```python
from build123d import *

# Parameters (mm, degrees)
SKETCH1_W                     = 17
SKETCH1_H                     = 39
SKETCH1_R                     = 1
SKETCH1_W_2                   = 12
SKETCH1_H_2                   = 23
SERVOBRACKET_DEPTH            = 2.5
SKETCH1_5_W                   = 2.5
SKETCH1_5_H                   = 10
SUPPORTLEGS_DEPTH             = 21.1
SKETCH2_W                     = 2
SKETCH2_H                     = 10
SUPPORTFOOT_DEPTH             = 5
BASEBOLTHOLE_START            = -3
SKETCH3_R                     = 1
BASEBOLTHOLE_DEPTH            = 25.6
SERVONUTSLOTS_DEPTH           = 1
BASENUTSLOTS_DEPTH            = 1
SKETCH6_W                     = 2.5
SKETCH6_H                     = 4
TUBEHOLDERBASE_DEPTH          = 12
SKETCH7_W                     = 4
SKETCH7_H                     = 1
TUBEHOLDERSTIFFENERRIBS_DEPTH = 30.6
SKETCH8_W                     = 1
SKETCH8_H                     = 1
SKETCH8_H_2                   = 0.25
TUBECLIPENTRANCES_DEPTH       = 2
SKETCH9_W                     = 1.5
SKETCH9_H                     = 1.5
TUBECLIPLOCKSLOT_DEPTH        = 0.6
TUBECLIPLOCKSLOT2_DEPTH       = 0.6
SUPPORTLEGEXTENSION_DEPTH     = 10.55
SKETCH8_4_W                   = 0.2
SKETCH8_4_H                   = 1.5
TUBECLIPLOCKCLEARANCE_DEPTH   = 0.5


with BuildPart() as part:
    # Sketch1 → ServoBracket (new body)
    with BuildSketch(Plane.XY):
        with Locations((0, 19.5)):
            Rectangle(SKETCH1_W, SKETCH1_H)
        with Locations((-3.5, 33.5)):
            Circle(SKETCH1_R, mode=Mode.SUBTRACT)
        with Locations((-3.5, 5.5)):
            Circle(SKETCH1_R, mode=Mode.SUBTRACT)
        with Locations((3.5, 5.5)):
            Circle(SKETCH1_R, mode=Mode.SUBTRACT)
        with Locations((3.5, 33.5)):
            Circle(SKETCH1_R, mode=Mode.SUBTRACT)
        with Locations((0, 19.5)):
            Rectangle(SKETCH1_W_2, SKETCH1_H_2, mode=Mode.SUBTRACT)
    extrude(amount=SERVOBRACKET_DEPTH)

    # Sketch1_5 → SupportLegs (add)
    with BuildSketch(Plane.XY):
        with Locations((-7.25, 19.5)):
            Rectangle(SKETCH1_5_W, SKETCH1_5_H)
        with Locations((7.25, 19.5)):
            Rectangle(SKETCH1_5_W, SKETCH1_5_H)
    extrude(amount=-SUPPORTLEGS_DEPTH)

    # Sketch2 → SupportFoot (add)
    with BuildSketch(Plane.ZY.offset(8.5)):
        with Locations((-20.1, 19.5)):
            Rectangle(SKETCH2_W, SKETCH2_H)
    supportfoot = extrude(amount=SUPPORTFOOT_DEPTH)

    # Sketch3 → BaseBoltHole (cut)
    with BuildSketch(Plane.XY.offset(-19.1).offset(BASEBOLTHOLE_START)):
        with Locations((-11, 19.5)):
            Circle(SKETCH3_R)
    basebolthole = extrude(amount=BASEBOLTHOLE_DEPTH, mode=Mode.SUBTRACT)

    # SupportFoot2: SupportFoot, BaseBoltHole across plane
    add(supportfoot.mirror(Plane(origin=(0, 0, 0), x_dir=(0, 0, 1), z_dir=(1, 0, 0))))
    add(basebolthole.mirror(Plane(origin=(0, 0, 0), x_dir=(0, 0, 1), z_dir=(1, 0, 0))), mode=Mode.SUBTRACT)

    # Sketch4 → ServoNutSlots (cut)
    with BuildSketch(Plane.XY.offset(2.5)):
        Polygon((-4.654700538, 7.5), (-2.345299462, 7.5), (-1.190598923, 5.5), (-2.345299462, 3.5), (-4.654700538, 3.5), (-5.809401077, 5.5), align=None)
        Polygon((-1.190598923, 33.5), (-2.345299462, 35.5), (-4.654700538, 35.5), (-5.809401077, 33.5), (-4.654700538, 31.5), (-2.345299462, 31.5), align=None)
        Polygon((2.345299462, 31.5), (1.190598923, 33.5), (2.345299462, 35.5), (4.654700538, 35.5), (5.809401077, 33.5), (4.654700538, 31.5), align=None)
        Polygon((4.654700538, 7.5), (2.345299462, 7.5), (1.190598923, 5.5), (2.345299462, 3.5), (4.654700538, 3.5), (5.809401077, 5.5), align=None)
    extrude(amount=-SERVONUTSLOTS_DEPTH, mode=Mode.SUBTRACT)

    # Sketch5 → BaseNutSlots (cut)
    with BuildSketch(Plane.XY.offset(-19.1)):
        Polygon((-11, 21.809401077), (-13, 20.654700538), (-13, 18.345299462), (-11, 17.190598923), (-9, 18.345299462), (-9, 20.654700538), align=None)
        Polygon((11, 21.809401077), (9, 20.654700538), (9, 18.345299462), (11, 17.190598923), (13, 18.345299462), (13, 20.654700538), align=None)
    extrude(amount=-BASENUTSLOTS_DEPTH, mode=Mode.SUBTRACT)

    # Sketch6 → TubeHolderBase (add)
    with BuildSketch(Plane.XY.offset(2.5)):
        with Locations((-7.25, 21.65)):
            Rectangle(SKETCH6_W, SKETCH6_H)
    tubeholderbase = extrude(amount=TUBEHOLDERBASE_DEPTH)

    # Sketch7 → TubeHolderStiffenerRibs (add)
    with BuildSketch(Plane.XY.offset(14.5)):
        with Locations((-10.5, 23.15)):
            Rectangle(SKETCH7_W, SKETCH7_H)
        with Locations((-10.5, 20.15)):
            Rectangle(SKETCH7_W, SKETCH7_H)
    tubeholderstiffenerribs = extrude(amount=-TUBEHOLDERSTIFFENERRIBS_DEPTH)

    # TubeHolder2: TubeHolderBase, TubeHolderStiffenerRibs across plane
    add(tubeholderbase.mirror(Plane.ZX.offset(13.8)))
    add(tubeholderstiffenerribs.mirror(Plane.ZX.offset(13.8)))

    # Sketch8 → TubeClipEntrances (cut)
    with BuildSketch(Plane.ZY.offset(8.5)):
        with Locations((11.1, 21.65)):
            Rectangle(SKETCH8_W, SKETCH8_H)
        with Locations((11.1, 22.275)):
            Rectangle(SKETCH8_W, SKETCH8_H_2)
        with Locations((11.1, 21.025)):
            Rectangle(SKETCH8_W, SKETCH8_H_2)
        with Locations((10.3, 6.575)):
            Rectangle(SKETCH8_W, SKETCH8_H_2)
        with Locations((10.3, 5.325)):
            Rectangle(SKETCH8_W, SKETCH8_H_2)
        with Locations((10.3, 5.95)):
            Rectangle(SKETCH8_W, SKETCH8_H)
    extrude(amount=-TUBECLIPENTRANCES_DEPTH, mode=Mode.SUBTRACT)

    # Sketch9 → TubeClipLockSlot (cut)
    with BuildSketch(Plane(origin=(0, 0, 11.6), x_dir=(-1, 0, 0), z_dir=(0, 0, -1))):
        with Locations((7.25, 21.65)):
            Rectangle(SKETCH9_W, SKETCH9_H)
    extrude(amount=-TUBECLIPLOCKSLOT_DEPTH, mode=Mode.SUBTRACT)

    # Sketch10 → TubeClipLockSlot2 (cut)
    with BuildSketch(Plane(origin=(0, 0, 10.8), x_dir=(-1, 0, 0), z_dir=(0, 0, -1))):
        Polygon((6.5, 5.45), (6.5, 5.2), (8, 5.2), (8, 6.7), (6.5, 6.7), align=None)
    extrude(amount=-TUBECLIPLOCKSLOT2_DEPTH, mode=Mode.SUBTRACT)

    # Sketch11 → SupportLegExtension (add)
    with BuildSketch(Plane.XZ.offset(-14.5)):
        Polygon((-6, 0), (-8.5, 0), (-8.5, -19.1), (-13.5, -19.1), (-13.5, -21.1), (-6, -21.1), align=None)
    extrude(amount=SUPPORTLEGEXTENSION_DEPTH)

    # Sketch8_4 → TubeClipLockClearance (cut)
    with BuildSketch(Plane.ZY.offset(8.5)):
        with Locations((10.9, 5.95)):
            Rectangle(SKETCH8_4_W, SKETCH8_4_H)
        with Locations((11.7, 21.65)):
            Rectangle(SKETCH8_4_W, SKETCH8_4_H)
    extrude(amount=-TUBECLIPLOCKCLEARANCE_DEPTH, mode=Mode.SUBTRACT)


solid = part.part
```
Work out the finished part from the listing and answer in its coordinate system (mm). A direction names the side the tool comes from. Give positions to 0.01 mm unless a question says otherwise; leave off trailing zeros. Loops run counter-clockwise (first coordinate to the right, second up) from the corner with the lowest first, then second, coordinate; pieces in that order, holes last. Notation, with made-up numbers: (-35, -15) -> (-13, -15) arc R16 cw to (-13, 12) -> close; hole circle Ø9 at (-34, 68). An arc over 180 degrees is marked (long way). Use CSV: the item, a comma, the result in double quotes.
1. The part is cut by section A-A (x = 3.5). Write down the section's boundary in (y, z).
Found:
outline,"(0, 0) -> (4.5, 0) -> (4.5, 1.5) -> (3.5, 1.5) -> (3.5, 2.5) -> (0, 2.5) -> close; (6.5, 0) -> (8, 0) -> (8, 2.5) -> (7.5, 2.5) -> (7.5, 1.5) -> (6.5, 1.5) -> close; (31, 0) -> (32.5, 0) -> (32.5, 1.5) -> (31.5, 1.5) -> (31.5, 2.5) -> (31, 2.5) -> close; (34.5, 0) -> (39, 0) -> (39, 2.5) -> (35.5, 2.5) -> (35.5, 1.5) -> (34.5, 1.5) -> close"
2. Straight lines are drawn through the part: line 1 (Y direction, x = -3.5, z = 0.5); line 2 (X direction, y = 19, z = -20); line 3 (Y direction, x = -11.5, z = 11.5). For each, find the intervals that lie inside material, in ascending order.
Found:
line 1,"0 to 4.5, 6.5 to 8, 31 to 32.5, 34.5 to 39"
line 2,"-13.5 to -13, -9 to -6, 6 to 9, 13 to 13.5"
line 3,"3.95 to 4.95, 6.95 to 7.95, 19.65 to 20.65, 22.65 to 23.65"
3. A tool of negligible diameter and unlimited length cuts with its end or side. For faces 5 (the flat face through (13, 19.5, -19.6)), 6 (the flat face through (-11, 23, -16.1)), 7 (the flat face through (9.7, 19.4, -21.1)), 8 (the flat face through (-10, 7.95, -1)), 9 (the flat face through (-7, 6, 11.4)), from which of +Z, -Z, +X, -X, +Y, -Y can it reach the whole face along a straight path? Write none if from no direction.
Found:
face 5,"+Z"
face 6,"-X, +Y, -Y"
face 7,"-Z, +X, -X, +Y, -Y"
face 8,"+Z, -X"
face 9,"none"
4. The mould has two halves that part along X. Classify faces 1 (the flat face through (3, 35.5, 2)), 2 (the flat face through (-6, 6, 8)), 3 (the flat face through (-13.5, 14, -20)), 4 (the flat face through (-3, 35.5, 2)): +X half, -X half, draft (parallel to the pull), parting line (faces both ways), or undercut.
Found:
face 1,"undercut"
face 2,"+X half"
face 3,"-X half"
face 4,"undercut"
5. The part is cut by section B-B (z = 5). Write down the section's boundary in (x, y), then the cut area to 3 significant figures.
Found:
outline,"(-12.5, 3.95) -> (-6, 3.95) -> (-6, 7.95) -> (-12.5, 7.95) -> (-12.5, 6.95) -> (-8.5, 6.95) -> (-8.5, 4.95) -> (-12.5, 4.95) -> close; (-12.5, 19.65) -> (-6, 19.65) -> (-6, 23.65) -> (-12.5, 23.65) -> (-12.5, 22.65) -> (-8.5, 22.65) -> (-8.5, 20.65) -> (-12.5, 20.65) -> close"
area,"36.0 mm^2"
6. The part is cut by section C-C (y = 11). Write down the section's boundary in (x, z).
Found:
outline,"(-13.5, -21.1) -> (-6, -21.1) -> (-6, 2.5) -> (-8.5, 2.5) -> (-8.5, -19.1) -> (-13.5, -19.1) -> close; (6, 0) -> (8.5, 0) -> (8.5, 2.5) -> (6, 2.5) -> close"
7. Flat-ended cylindrical pins translate along their axes: pin 1 Ø1 at (y, z) = (17, -14) entering from +X; pin 2 Ø11.5 at (x, y) = (-4, 31.5) entering from -Z; pin 3 Ø8 at (x, z) = (-5, -13) entering from -Y; pin 4 Ø1.8 at (x, y) = (-3.5, 5.5) entering from +Z. Find the tip coordinate at first contact, or state that the pin passes through.
Found:
pin 1,"x = 8.5"
pin 2,"z = 0"
pin 3,"y = 3.95"
pin 4,"through"
8. The part is cut by section D-D (x = -0.5). Write down the section's boundary in (y, z).
Found:
outline,"(0, 0) -> (8, 0) -> (8, 2.5) -> (0, 2.5) -> close; (31, 0) -> (39, 0) -> (39, 2.5) -> (31, 2.5) -> close"
